Source: CAD feature listing. Evaluate the final solid. Frame: model axes, mm. Round coordinates to 2 decimals unless told otherwise and drop trailing zeros. Write each loop counter-clockwise with the first axis right and the second up, starting at its lowest first coordinate (ties: lowest second). Pieces come first, ordered by that corner, then holes.
Autodesk Inventor part; units mm, degrees
ref_plane "Work Plane1" through (123.825, 0, 0) normal (1, 0, 0) x (0, 1, 0)
ref_plane "XZ Plane" through (0, 0, 0) normal (0, 1, 0) x (-1, 0, 0)
ref_plane "XY Plane" through (0, 0, 0) normal (0, 0, 1) x (1, 0, 0)
sketch "Sketch1" plane through (0, 0, 0) normal (0, 0, 1) x (1, 0, 0)
  circle A0 centre (0, 0) radius 127
  circle A1 centre (0, 0) radius 152.4
  dimension "d0" = 254
  dimension "d1" = 25.4
extrude "Extrusion1" add sketch "Sketch1" along normal mid plane 12.7
ref_plane "Work Plane1" through (123.825, 0, 0) normal (1, 0, 0) x (0, 1, 0)
sketch "Sketch3" plane through (123.825, 0, 0) normal (1, 0, 0) x (0, 1, 0)
  point P0 (0, 0)
  point P1 (0, 0)
hole "Hole1" at (123.825, 0, 0) at (123.825, 0, 0) direction (1, 0, 0) diameter 4.9784 end through all
pattern_circular "Circular Pattern1" count 3 over 360 about axis through (0, 0, -10) along (0, 0, 1) of "Hole1"
properties part number "ring_middle"
1) Section query B-B on y = 73.5. Return the cut outline in (x, z), then the cut area to 3 significant figures.
Taken from the geometry:
outline: (-133.5, -6.35) - (-103.57, -6.35) - (-103.57, 6.35) - (-133.5, 6.35) - close; (103.57, -6.35) - (133.5, -6.35) - (133.5, 6.35) - (103.57, 6.35) - close
area: 760 mm2
2) Material intervals for line 1 (Z direction, x = 135.75, y = 0); line 2 (Y direction, x = -0.5, z = -0.75); line 3 (Y direction, x = 41, z = -3), sorted ascending.
Taken from the geometry:
line 1: z = -6.35 to -2.49, 2.49 to 6.35
line 2: y = -152.4 to -127, 127 to 152.4
line 3: y = -146.78 to -120.2, 120.2 to 146.78
3) Section query C-C on z = 0. Return the cut outline in (x, y), then the cut area to 3 significant figures.
Taken from the geometry:
outline: (-78.35, -130.72) - (-65.64, -108.72) arc R127 cw to (-65.64, 108.72) - (-78.35, 130.72) arc R152.4 ccw to start; (-74.03, -133.21) arc R152.4 ccw to (152.38, -2.49) - (126.98, -2.49) arc R127 cw to (-61.33, -111.21) - close; (-74.03, 133.21) - (-61.33, 111.21) arc R127 cw to (126.98, 2.49) - (152.38, 2.49) arc R152.4 ccw to start
area: 21,900 mm2
4) Section query A-A on x = 0. Return the cut outline in (y, z).
Taken from the geometry:
outline: (-152.4, -6.35) - (-127, -6.35) - (-127, 6.35) - (-152.4, 6.35) - close; (127, -6.35) - (152.4, -6.35) - (152.4, 6.35) - (127, 6.35) - close
5) Contact query for flat-ended pins moving along their axis: P1, Ø1, axis at y = -6.5, z = 0.5, coming from the -X side; P2, Ø1.5, axis at y = -25.5, z = -4, coming from the -X side; P3, Ø5, axis at y = -88.5, z = -0.5, coming from the +X side. Output: stop coordinate, or through.
Taken from the geometry:
P1: stops at x = -152.28
P2: stops at x = -150.38
P3: stops at x = 125.82
6) Pull-direction query (X, two-part tool) for faces 1 (the face through (-120.94, 92.73, -0.09)), 2 (the face through (-57, 114, -6.35)), 3 (the face through (-69.11, -121.6, 2.3)); classes: released by +X, released by -X, zero draft, split by the parting line, or undercut.
Taken from the geometry:
face 1: split by the parting line
face 2: zero draft
face 3: undercut
